```python
from build123d import *

# Parameters (mm, degrees)
SKETCH1_R           = 7
SKETCH1_R_2         = 3
BOSS_EXTRUDE1_DEPTH = 14
SKETCH2_W           = 3
SKETCH2_H           = 2
SKETCH2_H_2         = 0.5


with BuildPart() as part:
    # Sketch1 → Boss-Extrude1 (new body)
    with BuildSketch(Plane(origin=(0, 0, 0), x_dir=(1, 0, 0), z_dir=(0, 1, 0))):
        with Locations(Location((0, 0, 0), (0, 0, 270))):
            Circle(SKETCH1_R)
        with Locations(Location((0, 0, 0), (0, 0, 270))):
            Circle(SKETCH1_R_2, mode=Mode.SUBTRACT)
    extrude(amount=BOSS_EXTRUDE1_DEPTH)

    # Sketch2 → Cut-Revolve1 (revolve, cut)
    with BuildSketch(Plane.XY, mode=Mode.PRIVATE) as cut_revolve1_sk:
        with Locations((5.5, 1)):
            Rectangle(SKETCH2_W, SKETCH2_H)
        with Locations((5.5, 13.75)):
            Rectangle(SKETCH2_W, SKETCH2_H_2)
    revolve(cut_revolve1_sk.sketch.rotate(Axis((0, 14, 0), (0, -1, 0)), 90), axis=Axis((0, 14, 0), (0, -1, 0)), mode=Mode.SUBTRACT)


solid = part.part
```
Geometry check sheet. Reference: the model listing, model coordinates, mm. A direction names the side the tool comes from. Give positions to 0.01 mm unless a question says otherwise; leave off trailing zeros. Loops run counter-clockwise (first coordinate to the right, second up) from the corner with the lowest first, then second, coordinate; pieces in that order, holes last. Notation, with made-up numbers: M 81,-29.5 L 122,-29.5 A21 ccw 122,-21.5 Z; hole C 2,-33 d4. An arc over 180 degrees is marked long. Answer as CSV lines item,"result".
Item 1: Material ranges on line 1 (X direction, y = 4.5, z = 0); line 2 (X direction, y = 8.25, z = 2.75); line 3 (Z direction, x = 0.5, y = 6.5), recorded low to high.
Values:
line 1,"x = -7 to -3, 3 to 7"
line 2,"x = -6.44 to -1.2, 1.2 to 6.44"
line 3,"z = -6.98 to -2.96, 2.96 to 6.98"
Item 2: Access from +Z, -Z, +X, -X, +Y, -Y to the whole of each face (thin tool, end or side, straight path). Record for faces 4 (the cylindrical face through (-6.834, 7.67, -1.517)), 5 (the cylindrical face through (3.905, 13.754, -0.867)), 6 (the flat face through (3, 2, -3)).
Values:
face 4,"+Y, -Y"
face 5,"+Y"
face 6,"-Y"
Item 3: Cross-section at D-D on x = -3.5. Record the cut outline in (y, z).
Values:
outline,"M 0,-1.94 L 2,-1.94 L 2,-6.06 L 13.5,-6.06 L 13.5,-1.94 L 14,-1.94 L 14,1.94 L 13.5,1.94 L 13.5,6.06 L 2,6.06 L 2,1.94 L 0,1.94 Z"
Item 4: Release check for a two-part mould opening along X. For faces 1 (the flat face through (3, 14, 1)), 2 (the cylindrical face through (0.9, 6.9, 2.86)), 3 (the cylindrical face through (3.905, 1.014, -0.867)) record: pulls with the +X half, pulls with the -X half, needs draft (parallel to the pull), parting line crosses it, or undercut.
Values:
face 1,"needs draft"
face 2,"undercut"
face 3,"parting line crosses it"
Item 5: Cross-section at B-B on x = 0. Record the cut outline in (y, z), and give its area (3 significant figures).
Values:
outline,"M 0,-4 L 2,-4 L 2,-7 L 13.5,-7 L 13.5,-4 L 14,-4 L 14,-3 L 0,-3 Z; M 0,3 L 14,3 L 14,4 L 13.5,4 L 13.5,7 L 2,7 L 2,4 L 0,4 Z"
area,"97.0 mm²"
Item 6: Depth check by flat-ended pin: P1, Ø3, axis at x = -3.5, y = 6, coming from the +Z side; P2, Ø1, axis at x = -3, y = 10, coming from the -Z side; P3, Ø3, axis at y = 2.5, z = -4, coming from the -X side; P4, Ø5.5, axis at x = 0, z = 0, coming from the +Y side. Enter the tip coordinate at first touch or a pass-through.
Values:
P1,"stops at z = 6.71"
P2,"stops at z = -6.54"
P3,"stops at x = -6.54"
P4,"passes through"
Item 7: Cross-section at C-C on y = 10. Record the cut outline in (x, z), and give its area (3 significant figures).
Values:
outline,"C 0,0 d14; hole C 0,0 d6"
area,"126 mm²"
Item 8: Cross-section at A-A on z = 0. Record the cut outline in (x, y), and give its area (3 significant figures).
Values:
outline,"M -7,2 L -4,2 L -4,0 L -3,0 L -3,14 L -4,14 L -4,13.5 L -7,13.5 Z; M 3,0 L 4,0 L 4,2 L 7,2 L 7,13.5 L 4,13.5 L 4,14 L 3,14 Z"
area,"97.0 mm²"
